from build123d import *

# Parameters (mm, degrees)
SKETCH1_W           = 60
SKETCH1_H           = 90
BOSS_EXTRUDE1_DEPTH = 20
CUT_EXTRUDE1_DEPTH  = 10
BOSS_EXTRUDE2_DEPTH = 10
SKETCH5_R           = 8.5
CUT_EXTRUDE2_DEPTH  = 143.214626533
FILLET1_R           = 10
SKETCH6_W           = 50
SKETCH6_H           = 15
CUT_EXTRUDE3_DEPTH  = 123.270192606
FILLET2_R           = 5


with BuildPart() as part:
    # Sketch1 → Boss-Extrude1 (new body)
    with BuildSketch(Plane(origin=(0, 0, 0), x_dir=(1, 0, 0), z_dir=(0, 1, 0))):
        Rectangle(SKETCH1_W, SKETCH1_H)
    extrude(amount=BOSS_EXTRUDE1_DEPTH)

    # Sketch3 → Cut-Extrude1 (cut)
    with BuildSketch(Plane(origin=(0, 20, 0), x_dir=(1, 0, 0), z_dir=(0, 1, 0))):
        with BuildLine():
            ThreePointArc((-20, 30), (-16.464466094, 31.464466094), (-15, 35))
            Line((-15, 35), (-20, 35))
            Line((-20, 35), (-20, 30))
        make_face()
        with BuildLine():
            Line((-20, 35), (-15, 35))
            ThreePointArc((-15, 35), (-23.535533906, 38.535533906), (-20, 30))
            Line((-20, 30), (-20, 35))
        make_face()
        with BuildLine():
            ThreePointArc((-20, 30), (-16.464466094, 31.464466094), (-15, 35))
            Line((-15, 35), (-20, 35))
            Line((-20, 35), (-20, 30))
        make_face()
        with BuildLine():
            Line((-20, 35), (-15, 35))
            ThreePointArc((-15, 35), (-23.535533906, 38.535533906), (-20, 30))
            Line((-20, 30), (-20, 35))
        make_face()
        with BuildLine():
            ThreePointArc((-20, -30), (-23.535533906, -38.535533906), (-15, -35))
            Line((-15, -35), (-20, -35))
            Line((-20, -35), (-20, -30))
        make_face()
        with BuildLine():
            Line((-20, -35), (-15, -35))
            ThreePointArc((-15, -35), (-16.464466094, -31.464466094), (-20, -30))
            Line((-20, -30), (-20, -35))
        make_face()
        with BuildLine():
            ThreePointArc((-20, -30), (-23.535533906, -38.535533906), (-15, -35))
            Line((-15, -35), (-20, -35))
            Line((-20, -35), (-20, -30))
        make_face()
        with BuildLine():
            Line((-20, -35), (-15, -35))
            ThreePointArc((-15, -35), (-16.464466094, -31.464466094), (-20, -30))
            Line((-20, -30), (-20, -35))
        make_face()
        with BuildLine():
            Line((15, -35), (20, -35))
            Line((20, -35), (20, -30))
            ThreePointArc((20, -30), (16.464466094, -31.464466094), (15, -35))
        make_face()
        with BuildLine():
            Line((20, -30), (20, -35))
            Line((20, -35), (15, -35))
            ThreePointArc((15, -35), (20, -40), (25, -35))
            ThreePointArc((25, -35), (23.535533906, -31.464466094), (20, -30))
        make_face()
        with BuildLine():
            Line((15, -35), (20, -35))
            Line((20, -35), (20, -30))
            ThreePointArc((20, -30), (16.464466094, -31.464466094), (15, -35))
        make_face()
        with BuildLine():
            Line((20, -30), (20, -35))
            Line((20, -35), (15, -35))
            ThreePointArc((15, -35), (20, -40), (25, -35))
            ThreePointArc((25, -35), (23.535533906, -31.464466094), (20, -30))
        make_face()
        with BuildLine():
            ThreePointArc((15, 35), (16.464466094, 31.464466094), (20, 30))
            Line((20, 30), (20, 35))
            Line((20, 35), (15, 35))
        make_face()
        with BuildLine():
            Line((20, 35), (20, 30))
            ThreePointArc((20, 30), (23.535533906, 31.464466094), (25, 35))
            ThreePointArc((25, 35), (20, 40), (15, 35))
            Line((15, 35), (20, 35))
        make_face()
        with BuildLine():
            ThreePointArc((15, 35), (16.464466094, 31.464466094), (20, 30))
            Line((20, 30), (20, 35))
            Line((20, 35), (15, 35))
        make_face()
        with BuildLine():
            Line((20, 35), (20, 30))
            ThreePointArc((20, 30), (23.535533906, 31.464466094), (25, 35))
            ThreePointArc((25, 35), (20, 40), (15, 35))
            Line((15, 35), (20, 35))
        make_face()
    extrude(amount=-CUT_EXTRUDE1_DEPTH, mode=Mode.SUBTRACT)

    # Sketch4 → Boss-Extrude2 (add)
    with BuildSketch(Plane.XY.offset(45)):
        with BuildLine():
            Line((-30, 0), (-30, -55))
            ThreePointArc((-30, -55), (0, -85), (30, -55))
            Line((30, -55), (30, 0))
            Line((30, 0), (30, 20))
            Line((30, 20), (-30, 20))
            Line((-30, 20), (-30, 0))
        make_face()
    boss_extrude2 = extrude(amount=BOSS_EXTRUDE2_DEPTH)

    # Mirror1: Boss-Extrude2 across plane
    add(boss_extrude2.mirror(Plane.XY))

    # Sketch5 → Cut-Extrude2 (cut, through all)
    with BuildSketch(Plane.XY.offset(55)):
        with Locations((0, -55)):
            Circle(SKETCH5_R)
    extrude(amount=-CUT_EXTRUDE2_DEPTH, mode=Mode.SUBTRACT)

    # Fillet1
    fillet1_edges = [part.edges().sort_by_distance(p)[0] for p in [
        (0, 20, 55),
        (0, 20, -55),
    ]]
    fillet(fillet1_edges, radius=FILLET1_R)

    # Sketch6 → Cut-Extrude3 (cut, through all)
    with BuildSketch(Plane(origin=(0, 20, 0), x_dir=(1, 0, 0), z_dir=(0, 1, 0))):
        with Locations((0, -17.5)):
            Rectangle(SKETCH6_W, SKETCH6_H)
    extrude(amount=-CUT_EXTRUDE3_DEPTH, mode=Mode.SUBTRACT)

    # Fillet2
    fillet2_edges = [part.edges().sort_by_distance(p)[0] for p in [
        (-25, 0, 17.5),
        (25, 0, 17.5),
    ]]
    fillet(fillet2_edges, radius=FILLET2_R - 0.0001)  # a hair under: the kernel refuses the full size


solid = part.part
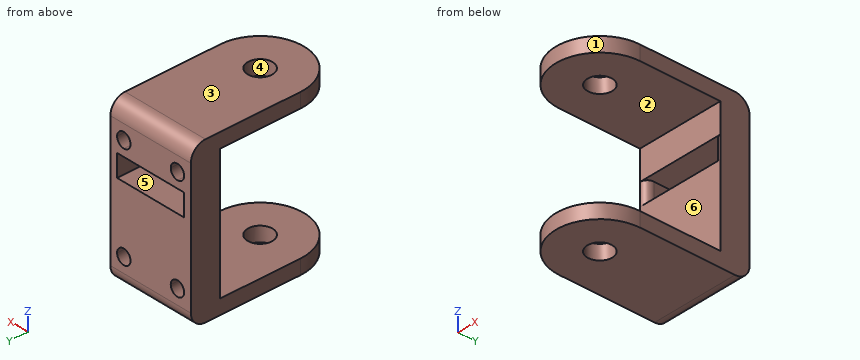
Could you check a few things on this model? Use its own coordinates, in mm. Face numbers are marked on the shaded views. A direction names the side the tool comes from. Round coordinates to 2 decimals unless told otherwise and drop trailing zeros. Order: outer loops, then holes, each group sorted by start corner. A loop starts at its lowest first (then second) coordinate and runs counter-clockwise, first axis right, second up.
Q1. I'm going to push flat-ended pins straight in: P1, Ø9, axis at x = -20, z = -35, coming from the +Y side; P2, Ø6, axis at x = 5.5, y = 13.5, coming from the +Z side; P3, Ø10, axis at x = 0, y = -55, coming from the +Z side; P4, Ø6, axis at x = 8.5, y = 14.5, coming from the -Z side. Where does each tip first touch, or does it pass through?
Geometry says:
P1: stops at y = 10
P2: stops at z = 54.99
P3: passes through
P4: stops at z = -54.89
Q2. Which directions (+Z, -Z, +X, -X, +Y, -Y) give clear straight access to the entire face, cutting with the end or side of a thin tool? Please do the marked faces 1 and 2.
Geometry says:
face 1: +Z, -Z, -Y
face 2: +X, -X, -Y
Q3. Imagine slicing it at B-B, the plane x = 10.5. List the corners of the cut face in (y, z) for me, then the cut area to 3 significant figures.
Geometry says:
outline: (-83.1, -55) - (10, -55) arc R10 ccw to (20, -45) - (20, 10) - (0, 10) - (0, -45) - (-83.1, -45) - close; (-83.1, 45) - (0, 45) - (0, 25) - (20, 25) - (20, 45) arc R10 ccw to (10, 55) - (-83.1, 55) - close
area: 3,520 mm2
Q4. Imagine slicing it at D-D, the plane z = 4.5. List the corners of the cut face in (x, y) for me.
Geometry says:
outline: (-30, 0) - (30, 0) - (30, 20) - (-30, 20) - close
Q5. Please list where these lines run through material, in increasing order: probe 1 along X at (y, z) = (15, -35); probe 2 along Z at (x, y) = (19.5, -28.5); probe 3 along Z at (x, y) = (-20, 16).
Geometry says:
probe 1: x = -30 to -25, -15 to 15, 25 to 30
probe 2: z = -55 to -45, 45 to 55
probe 3: z = -53 to -40, -30 to 10, 25 to 30, 40 to 53
Q6. Thinking about a two-plate mould opening in Z: for the marked faces 3, 4, 5 and 6, which applies, released by +Z, released by -Z, zero draft, split by the parting line, or undercut?
Geometry says:
face 3: released by +Z
face 4: zero draft
face 5: undercut
face 6: undercut
Q7. Imagine slicing it at A-A, the plane y = -22. List the corners of the cut face in (x, z) for me.
Geometry says:
outline: (-30, -55) - (30, -55) - (30, -45) - (-30, -45) - close; (-30, 45) - (30, 45) - (30, 55) - (-30, 55) - close
Q8. Imagine slicing it at C-C, the plane y = -50.5. List the corners of the cut face in (x, z) for me, then the cut area to 3 significant figures.
Geometry says:
outline: (-30, -55) - (-7.21, -55) - (-7.21, -45) - (-30, -45) - close; (-30, 45) - (-7.21, 45) - (-7.21, 55) - (-30, 55) - close; (7.21, -55) - (30, -55) - (30, -45) - (7.21, -45) - close; (7.21, 45) - (30, 45) - (30, 55) - (7.21, 55) - close
area: 912 mm2
